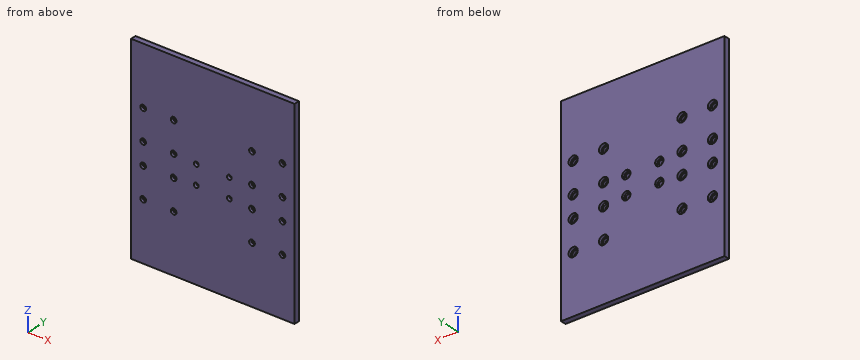
```python
from build123d import *

# Parameters (mm, degrees)
SKETCH1_W        = 187.8
SKETCH1_H        = 228.6
EXTRUSION1_DEPTH = 6.35
HOLE4_D          = 6.6
HOLE5_D          = 5.5
HOLE6_D          = 10.6
HOLE6_DEPTH      = 3.3
HOLE7_D          = 9.6
HOLE7_DEPTH      = 2.75


with BuildPart() as part:
    # Sketch1 → Extrusion1 (new body)
    with BuildSketch(Plane(origin=(0, 0, 0), x_dir=(-1, 0, 0), z_dir=(0, 1, 0))):
        Rectangle(SKETCH1_W, SKETCH1_H)
    extrude(amount=EXTRUSION1_DEPTH)

    # Hole4 (through all)
    with Locations(Plane(origin=(0, 6.35, 0), x_dir=(1, 0, 0), z_dir=(0, 1, 0))):
        with Locations((-80.0034, 12.5), (-80.0034, 47.5), (-80.0034, -12.5), (-80.0034, -47.5), (-45.0034, -12.5), (-45.0034, -47.5), (-45.0034, 12.5), (-45.0034, 47.5), (80.0034, 47.5), (80.0034, 12.5), (80.0034, -12.5), (80.0034, -47.5), (45.0034, -47.5), (45.0034, -12.5), (45.0034, 12.5), (45.0034, 47.5)):
            Hole(HOLE4_D / 2)

    # Hole5 (through all)
    with Locations(Plane(origin=(0, 6.35, 0), x_dir=(1, 0, 0), z_dir=(0, 1, 0))):
        with Locations((-19, 11), (19, 11), (-19, -11), (19, -11)):
            Hole(HOLE5_D / 2)

    # Hole6
    with Locations(Plane(origin=(-80.0034, 6.35, -47.5), x_dir=(0, 0, -1), z_dir=(0, 1, 0))):
        with Locations((0, 0), (0, -35), (-35, -35), (-35, 0), (-60, 0), (-60, -35), (-95, -35), (-95, 0), (-95, -160.0068), (-60, -160.0068), (0, -160.0068), (-35, -160.0068), (0, -125.0068), (-35, -125.0068), (-95, -125.0068), (-60, -125.0068)):
            Hole(HOLE6_D / 2, depth=HOLE6_DEPTH)

    # Hole7
    with Locations(Plane(origin=(-19, 6.35, -11), x_dir=(0, 0, -1), z_dir=(0, 1, 0))):
        with Locations((0, 0), (0, -38), (-22, -38), (-22, 0)):
            Hole(HOLE7_D / 2, depth=HOLE7_DEPTH)


solid = part.part
```
Geometry check sheet. Reference: the model listing, model coordinates, mm. Give positions to 0.01 mm unless a question says otherwise; leave off trailing zeros. Order: outer loops, then holes, each group sorted by start corner. A loop starts at its lowest first (then second) coordinate and runs counter-clockwise, first axis right, second up. Notation, with made-up numbers: (85.5, 7) - (108.5, 7) arc R10 ccw to (108.5, 22) - close; hole circle Ø5 at (87.25, -9). An arc over 180 degrees is marked (long way). Write item = value, one per line. Start each with the question number.
1) Section check B-B (z = 47.5). Count the separate pieces of the cut face and the enclosed holes in it, then the cut area to 3 significant figures.
2) Gauge pin test, flat ends, axial feed: pin 1 Ø6.5 at (x, z) = (-80, 47.5) entering from +Y; pin 2 Ø8.5 at (x, z) = (-45, 47.5) entering from +Y; pin 3 Ø10.5 at (x, z) = (17, 13.5) entering from +Y. Record the tip position at first contact, or that the pin passes through.
3) Scan lines: L1, parallel to Z at x = -45.5, y = 5.25; L2, parallel to X at y = 3.5, z = -47.5; L3, parallel to X at y = 2.3, z = 47.5. Record each from-to range of solid material in increasing order.
4) Section check A-A (x = -19). Enter the section's corners in (y, z), then the cut area to 3 significant figures.
Geometry check:
q1.separate_pieces = 5
q1.enclosed_holes = 0
q1.area = 972 mm2
q2.pin_1 = through
q2.pin_2 = 3.05
q2.pin_3 = 6.35
q3.L1 = -114.3 to -52.78, -42.22 to -17.78, -7.22 to 7.22, 17.78 to 42.22, 52.78 to 114.3
q3.L2 = -93.9 to -85.3, -74.7 to -50.3, -39.7 to 39.7, 50.3 to 74.7, 85.3 to 93.9
q3.L3 = -93.9 to -83.3, -76.7 to -48.3, -41.7 to 41.7, 48.3 to 76.7, 83.3 to 93.9
q4.outline = (0, -114.3) - (6.35, -114.3) - (6.35, -15.8) - (3.6, -15.8) - (3.6, -13.75) - (0, -13.75) - close; (0, -8.25) - (3.6, -8.25) - (3.6, -6.2) - (6.35, -6.2) - (6.35, 6.2) - (3.6, 6.2) - (3.6, 8.25) - (0, 8.25) - close; (0, 13.75) - (3.6, 13.75) - (3.6, 15.8) - (6.35, 15.8) - (6.35, 114.3) - (0, 114.3) - close
q4.area = 1,360 mm2
